Model file for the job. Use its own axes, mm. A direction names the side the tool comes from. Coordinates: 2 decimals unless noted, no trailing zeros. Order: outer loops, then holes, each group sorted by start corner. A loop starts at its lowest first (then second) coordinate and runs counter-clockwise, first axis right, second up. Notation, with made-up numbers: (21, 42) -> (29, 42) arc R23 ccw to (29, 70) -> close; hole circle Ø9 at (81, 82). An arc over 180 degrees is marked (long way). Use CSV: the item, a comma, the result in double quotes. Start each with the question number.
(1) Cut at A-A on x = 0. Write the cut outline in (y, z).
(2) Cut at D-D on x = -9. Write the cut outline in (y, z), plus the area to 3 significant figures.
(3) Cut at B-B on z = -122.5. Write the cut outline in (x, y).
(4) Tool access for faces 1 (the flat face through (0, 197, -47.354)), 2 (the flat face through (29.35, 197, -81)), 3 (the cylindrical face through (-17.717, 196.501, -54.052)): list every direction of +Z, -Z, +X, -X, +Y, -Y with a clear straight run to the whole face (end or side of a thin tool).
(5) Probe L1, parallel to X at y = 199, z = -72 (3 decimals); L2, parallel to X at y = 196.5, z = -137; L3, parallel to Z at x = -22.5, y = 197.25. List the from-to ranges inside material, lowest first.
(6) Pin check, flat tips, straight feed: pin 1 Ø5 at (x, z) = (23, -53.7) entering from -Y; pin 2 Ø2 at (y, z) = (196.5, -85) entering from -X; pin 3 Ø2 at (y, z) = (195, -116.5) entering from -X; pin 4 Ø1.9 at (x, y) = (4, 196) entering from -Z. Stop position of each tip, or through.
(7) Pull direction X, two halves, no side cores. Call faces 4 (the cylindrical face through (-17.652, 196.501, -89.421)), 5 (the flat face through (-29.35, 197, -82)), 6 (the cylindrical face through (0.865, 196.501, -167.693)), 7 (the flat face through (0, 197, -90.609)): pulls with the +X half, pulls with the -X half, needs draft (parallel to the pull), parting line crosses it, or undercut.
(8) Cut at C-C on y = 195.5. Give the number of separate pieces and of enclosed holes in the cut face, plus the area to 3 significant figures.
```python
from build123d import *

# Parameters (mm, degrees)
SKETCH1_R           = 2.75
SKETCH1_R_2         = 15.875
SKETCH1_R_3         = 2
BOSS_EXTRUDE1_DEPTH = 6.35
SKETCH2_R           = 3.175
CUT_EXTRUDE1_DEPTH  = 171.942179124


with BuildPart() as part:
    # Sketch1 → Boss-Extrude1 (new body)
    with BuildSketch(Plane.XZ.offset(-199.631527043)):
        with BuildLine():
            Line((-29.35, -47.354073009), (29.35, -47.354073009))
            Line((29.35, -47.354073009), (29.35, -116.366676692))
            ThreePointArc((29.35, -116.366676692), (29.697848179, -120.5559116), (30.731865285, -124.630404955))
            ThreePointArc((30.731865285, -124.630404955), (0, -167.704073009), (-30.731865285, -124.630404955))
            ThreePointArc((-30.731865285, -124.630404955), (-29.697848179, -120.5559116), (-29.35, -116.366676692))
            Line((-29.35, -116.366676692), (-29.35, -47.354073009))
        make_face()
        with Locations(Location((-23, -71.704073009, 0), (0, 0, 270))):
            Circle(SKETCH1_R, mode=Mode.SUBTRACT)
        with Locations(Location((-23, -53.704073009, 0), (0, 0, 270))):
            Circle(SKETCH1_R, mode=Mode.SUBTRACT)
        with Locations(Location((23, -53.704073009, 0), (0, 0, 270))):
            Circle(SKETCH1_R, mode=Mode.SUBTRACT)
        with Locations(Location((23, -71.704073009, 0), (0, 0, 270))):
            Circle(SKETCH1_R, mode=Mode.SUBTRACT)
        with Locations(Location((0, -135.204073009, 0), (0, 0, 270))):
            Circle(SKETCH1_R_2, mode=Mode.SUBTRACT)
        with Locations(Location((-22.20000005, -135.204073009, 0), (0, 0, 270))):
            Circle(SKETCH1_R_3, mode=Mode.SUBTRACT)
        with Locations(Location((0, -113.004072959, 0), (0, 0, 270))):
            Circle(SKETCH1_R_3, mode=Mode.SUBTRACT)
        with Locations(Location((22.20000005, -135.204073009, 0), (0, 0, 270))):
            Circle(SKETCH1_R_3, mode=Mode.SUBTRACT)
        with Locations(Location((0, -157.404073059, 0), (0, 0, 270))):
            Circle(SKETCH1_R_3, mode=Mode.SUBTRACT)
        with BuildLine():
            Line((-14.739402973, -52.799073011), (14.739402973, -52.799073011))
            ThreePointArc((14.739402973, -52.799073011), (17.684924877, -54.019148132), (18.905, -56.964670036))
            Line((18.905, -56.964670036), (18.905, -86.443475982))
            ThreePointArc((18.905, -86.443475982), (17.684924878, -89.388997884), (14.739402976, -90.609073006))
            Line((14.739402976, -90.609073006), (-14.739402973, -90.609073006))
            ThreePointArc((-14.739402973, -90.609073006), (-17.684924877, -89.388997886), (-18.905, -86.443475982))
            Line((-18.905, -86.443475982), (-18.905, -56.964670036))
            ThreePointArc((-18.905, -56.964670036), (-17.684924877, -54.019148132), (-14.739402973, -52.799073011))
        make_face(mode=Mode.SUBTRACT)
    extrude(amount=BOSS_EXTRUDE1_DEPTH)

    # Sketch2 → Cut-Extrude1 (cut, through all)
    with BuildSketch(Plane.XZ.offset(-193.281527043)):
        with Locations(Location((-22.225, -106.629073009, 0), (0, 0, 270))):
            Circle(SKETCH2_R)
    extrude(amount=-CUT_EXTRUDE1_DEPTH, mode=Mode.SUBTRACT)


solid = part.part
```
Outcome:
1,outline,"(193.28, -167.7) -> (199.63, -167.7) -> (199.63, -159.4) -> (193.28, -159.4) -> close; (193.28, -155.4) -> (199.63, -155.4) -> (199.63, -151.08) -> (193.28, -151.08) -> close; (193.28, -119.33) -> (199.63, -119.33) -> (199.63, -115) -> (193.28, -115) -> close; (193.28, -111) -> (199.63, -111) -> (199.63, -90.61) -> (193.28, -90.61) -> close; (193.28, -52.8) -> (199.63, -52.8) -> (199.63, -47.35) -> (193.28, -47.35) -> close"
2,outline,"(193.28, -166.43) -> (199.63, -166.43) -> (199.63, -148.28) -> (193.28, -148.28) -> close; (193.28, -122.13) -> (199.63, -122.13) -> (199.63, -90.61) -> (193.28, -90.61) -> close; (193.28, -52.8) -> (199.63, -52.8) -> (199.63, -47.35) -> (193.28, -47.35) -> close"
2,area,"350 mm2"
3,outline,"(-30.1, 193.28) -> (-9.52, 193.28) -> (-9.52, 199.63) -> (-30.1, 199.63) -> close; (9.52, 193.28) -> (30.1, 193.28) -> (30.1, 199.63) -> (9.52, 199.63) -> close"
4,face 1,"+Z, +X, -X, +Y, -Y"
4,face 2,"+Z, +X, +Y, -Y"
4,face 3,"+Y, -Y"
5,L1,"-29.35 to -25.734, -20.266 to -18.905, 18.905 to 20.266, 25.734 to 29.35"
5,L2,"-32.45 to -23.08, -21.32 to -15.77, 15.77 to 21.32, 23.08 to 32.45"
5,L3,"-158.66 to -137.18, -133.23 to -109.79, -103.47 to -74.41, -69 to -56.41, -51 to -47.35"
6,pin 1,"through"
6,pin 2,"x = -29.35"
6,pin 3,"x = -29.38"
6,pin 4,"z = -167.56"
7,face 4,"undercut"
7,face 5,"pulls with the -X half"
7,face 6,"parting line crosses it"
7,face 7,"undercut"
8,separate pieces,"1"
8,enclosed holes,"11"
8,area,"4,490 mm2"
